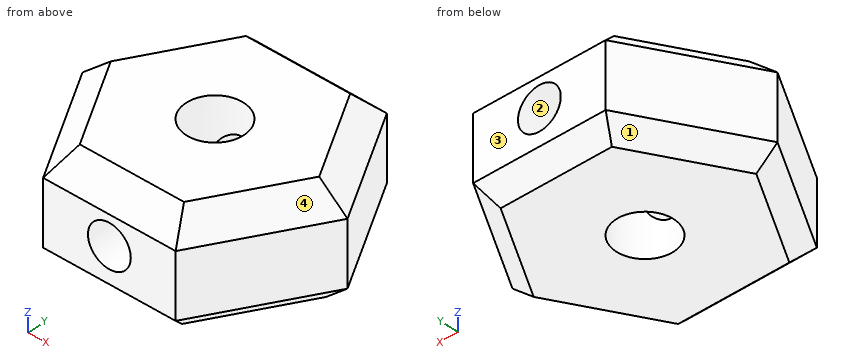
```python
from build123d import *

# Parameters (mm, degrees)
SKETCH1_R           = 1.9
BOSS_EXTRUDE1_DEPTH = 7
SKETCH2_R           = 1.4
CUT_EXTRUDE1_DEPTH  = 16
CHAMFER1_SIZE       = 1.6
CHAMFER2_SIZE       = 1.2


with BuildPart() as part:
    # Sketch1 → Boss-Extrude1 (new body)
    with BuildSketch(Plane.XY):
        Polygon((8.660254038, 0), (4.330127019, 7.5), (-4.330127019, 7.5), (-8.660254038, 0), (-4.330127019, -7.5), (4.330127019, -7.5), align=None)
        Circle(SKETCH1_R, mode=Mode.SUBTRACT)
    extrude(amount=BOSS_EXTRUDE1_DEPTH)

    # Sketch2 → Cut-Extrude1 (cut, through all)
    with BuildSketch(Plane.XZ.offset(7.5)):
        with Locations((0, 3.5)):
            Circle(SKETCH2_R)
    extrude(amount=-CUT_EXTRUDE1_DEPTH, mode=Mode.SUBTRACT)

    # Chamfer1
    chamfer1_edges = [part.edges().sort_by_distance(p)[0] for p in [
        (0, 7.5, 7),
        (-6.495190528, 3.75, 7),
        (-6.495190528, -3.75, 7),
        (0, -7.5, 7),
        (6.495190528, -3.75, 7),
        (6.495190528, 3.75, 7),
    ]]
    chamfer(chamfer1_edges, length=CHAMFER1_SIZE)

    # Chamfer2
    chamfer2_edges = [part.edges().sort_by_distance(p)[0] for p in [
        (0, -7.5, 0),
        (-6.495190528, -3.75, 0),
        (-6.495190528, 3.75, 0),
        (0, 7.5, 0),
        (6.495190528, 3.75, 0),
        (6.495190528, -3.75, 0),
    ]]
    chamfer(chamfer2_edges, length=CHAMFER2_SIZE)


solid = part.part
```
Geometry: final body of the model. Coordinates: model frame, mm. Face numbers are marked on the shaded views. Round coordinates to 2 decimals unless told otherwise and drop trailing zeros. Write each loop counter-clockwise with the first axis right and the second up, starting at its lowest first coordinate (ties: lowest second). Pieces come first, ordered by that corner, then holes. Notation, with made-up numbers: M 84,-35 L 131,-35 A33 cw 131,-7 Z; hole C -12.5,-27.75 d8. An arc over 180 degrees is marked long. Answer in a Markdown table with one row per item. Add a question column.
(1) Ray query, L1, parallel to Z at x = 0, y = -3.75; L2, parallel to Y at x = 0.5, z = 1.5; L3, parallel to X at y = -3, z = 3.5. Return the intervals inside material, ascending.
(2) Contact query for a flat-ended pin moving along its axis: pin 1 (2 mm diameter, centred on y = -0.5, z = 3.5, fed in from -X). Output: stop coordinate, or through.
(3) Cut plane A-A, the plane x = 0. Return the cut outline in (y, z), then the cut area to 3 significant figures.
(4) Cut plane D-D, the plane y = -4. Return the cut outline in (x, z), then the cut area to 3 significant figures.
(5) Cut plane B-B, the plane z = 3.5. Return the cut outline in (x, y).
(6) Cut plane C-C, the plane y = 0.5. Return the cut outline in (x, z).
(7) Draft query along Z for the marked faces 1, 2, 3 and 4. Return one class per face: pulls with the +Z half, pulls with the -Z half, needs draft (parallel to the pull), parting line crosses it, or undercut.
Established:
| question | item | result |
|---|---|---|
| 1 | L1 | 0 to 2.1, 4.9 to 7 |
| 1 | L2 | -7.5 to -1.83, 1.83 to 7.5 |
| 1 | L3 | -6.93 to -1.4, 1.4 to 6.93 |
| 2 | pin 1 | x = -8.66 |
| 3 | outline | M -7.5,1.2 L -6.3,0 L -1.9,0 L -1.9,2.1 L -7.5,2.1 Z; M -7.5,4.9 L -1.9,4.9 L -1.9,7 L -5.9,7 L -7.5,5.4 Z; M 1.9,0 L 6.3,0 L 7.5,1.2 L 7.5,2.1 L 1.9,2.1 Z; M 1.9,4.9 L 7.5,4.9 L 7.5,5.4 L 5.9,7 L 1.9,7 Z |
| 3 | area | 43.0 mm² |
| 4 | outline | M -6.35,1.2 L -4.97,0 L 4.97,0 L 6.35,1.2 L 6.35,5.4 L 4.5,7 L -4.5,7 L -6.35,5.4 Z; hole C 0,3.5 d2.8 |
| 4 | area | 78.1 mm² |
| 5 | outline | M -8.66,0 L -4.33,-7.5 L -1.4,-7.5 L -1.4,-1.28 A1.9 cw -1.4,1.28 L -1.4,7.5 L -4.33,7.5 Z; M 1.4,-7.5 L 4.33,-7.5 L 8.66,0 L 4.33,7.5 L 1.4,7.5 L 1.4,1.28 A1.9 cw 1.4,-1.28 Z |
| 6 | outline | M -8.37,1.2 L -6.99,0 L -1.83,0 L -1.83,7 L -6.52,7 L -8.37,5.4 Z; M 1.83,0 L 6.99,0 L 8.37,1.2 L 8.37,5.4 L 6.52,7 L 1.83,7 Z |
| 7 | face 1 | pulls with the -Z half |
| 7 | face 2 | undercut |
| 7 | face 3 | needs draft |
| 7 | face 4 | pulls with the +Z half |
